Could you check a few things on this model? Use its own coordinates, in mm. Face numbers are marked on the shaded views. Coordinates: 2 decimals unless noted, no trailing zeros. Loops run counter-clockwise (first coordinate to the right, second up) from the corner with the lowest first, then second, coordinate; pieces in that order, holes last.
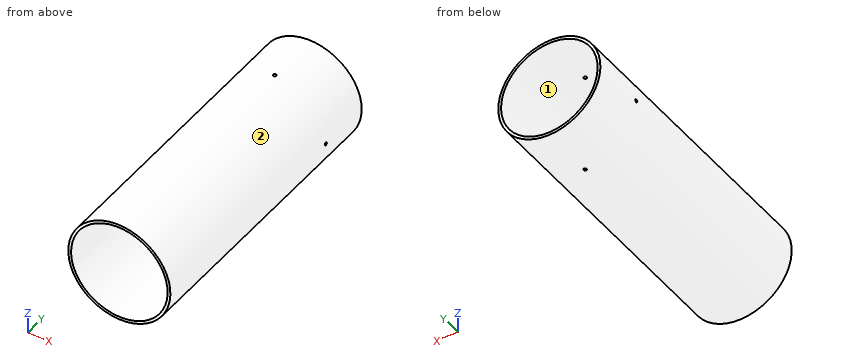
from build123d import *

# Parameters (mm, degrees)
SKETCH1_R               = 53.721
SKETCH1_R_2             = 50.8
TUBE_EXTRUSION_DEPTH    = 304.8
CUT_EXTRUDE1_REACH      = 329.617
CUT_EXTRUDE1_END_RADIUS = 50.8
SKETCH2_R               = 1.6383
CIRPATTERN1_COUNT       = 4


with BuildPart() as part:
    # Sketch1 → Tube Extrusion (new body)
    with BuildSketch(Plane(origin=(0, 0, 0), x_dir=(1, 0, 0), z_dir=(0, 1, 0))):
        with Locations(Location((0, 0, 0), (0, 0, 90))):
            Circle(SKETCH1_R)
        with Locations(Location((0, 0, 0), (0, 0, 90))):
            Circle(SKETCH1_R_2, mode=Mode.SUBTRACT)
    extrude(amount=TUBE_EXTRUSION_DEPTH)

    # Cut-Extrude1: up to this cylinder (the profile starts outside it)
    cut_extrude1_end = Plane(origin=(0, 247.65, 0), z_dir=(0, -1, 0)) * Cylinder(CUT_EXTRUDE1_END_RADIUS, 761.834, mode=Mode.PRIVATE)
    # Sketch2 → Cut-Extrude1 (cut, up to the surface)
    with BuildSketch(Plane(origin=(53.721, 0, 0), x_dir=(0, 0, -1), z_dir=(1, 0, 0)), mode=Mode.PRIVATE) as cut_extrude1_sk1:
        with Locations((0, 247.65)):
            Circle(SKETCH2_R)
    cut_extrude1_tool1 = extrude(cut_extrude1_sk1.sketch, amount=-CUT_EXTRUDE1_REACH, mode=Mode.PRIVATE) - cut_extrude1_end
    cut_extrude1 = cut_extrude1_tool1.solids().sort_by_distance((53.721, 247.65, 0))[0]
    add(cut_extrude1, mode=Mode.SUBTRACT)

    # CirPattern1: Cut-Extrude1 ×4 about axis
    cirpattern1_axis = Axis((0, 304.8, 0), (0, -1, 0))
    for i in range(1, CIRPATTERN1_COUNT):
        add(cut_extrude1.rotate(cirpattern1_axis, i * 360 / CIRPATTERN1_COUNT), mode=Mode.SUBTRACT)


solid = part.part
(1) Imagine slicing it at C-C, the plane y = 33. Write out the boundary of the cut face in (x, z).
Answers:
outline: circle Ø107.44 at (0, 0); hole circle Ø101.6 at (0, 0)
(2) For pin 1 (2 mm diameter, centred on x = -5, y = 67, fed in from -Z); pin 2 (2 mm diameter, centred on x = -29, y = 109, fed in from +Z); pin 3 (8 mm diameter, centred on y = 240, z = 14, fed in from -X), each with a flat end and sliding along its axis, tell me the tip position at first contact or that it passes through.
Answers:
pin 1: stops at z = -53.57
pin 2: stops at z = 45.85
pin 3: stops at x = -52.78
(3) Imagine slicing it at B-B, the plane x = 15. Write out the boundary of the cut face in (y, z), and give its area (3 significant figures).
Answers:
outline: (0, -51.58) - (304.8, -51.58) - (304.8, -48.53) - (0, -48.53) - close; (0, 48.53) - (304.8, 48.53) - (304.8, 51.58) - (0, 51.58) - close
area: 1,860 mm2
(4) Imagine slicing it at A-A, the plane z = -4.5. Write out the boundary of the cut face in (x, y).
Answers:
outline: (-53.53, 0) - (-50.6, 0) - (-50.6, 304.8) - (-53.53, 304.8) - close; (50.6, 0) - (53.53, 0) - (53.53, 304.8) - (50.6, 304.8) - close
(5) We'd pull the mould along Z, two halves only. Please class the marked faces 1 and 2: +Z half, -Z half, draft (parallel to the pull), parting line (faces both ways), or undercut.
Answers:
face 1: undercut
face 2: parting line
(6) I need wall thicknesses on probe 1 along Y at (x, z) = (52.75, 0); probe 2 along Z at (x, y) = (1, 135); probe 3 along X at (y, z) = (101, 0). Which ranges of each line are inside material? Lowest first, please.
Answers:
probe 1: y = 0 to 246.01, 249.29 to 304.8
probe 2: z = -53.71 to -50.79, 50.79 to 53.71
probe 3: x = -53.72 to -50.8, 50.8 to 53.72
